For this review, take the finished solid that the model builds, in its own axes (mm). A direction names the side the tool comes from. Give positions to 0.01 mm unless a question says otherwise; leave off trailing zeros. Loops run counter-clockwise (first coordinate to the right, second up) from the corner with the lowest first, then second, coordinate; pieces in that order, holes last. Notation, with made-up numbers: (-13.5, -14) -> (39.5, -14) arc R24 ccw to (39.5, 8) -> close; hole circle Ø4 at (84, -24.5). An arc over 180 degrees is marked (long way). One line per question, with ' | ' between items. Start each with the question number.
(1) Consider section D-D (x = -9). Write out the cut boundary in (y, z).
(2) Consider section C-C (y = 0.25). Give the number of separate pieces and of enclosed holes in the cut face, and give its area (3 significant figures).
(3) Draft analysis for pull direction X (two halves, no side actions). For faces 1 (the flat face through (-17, 0, 0)), 2 (the cylindrical face through (-12, 0, -26)), 3 (the cylindrical face through (16.1, -0.02, -28.14)), state which applies: +X half, -X half, draft (parallel to the pull), parting line (faces both ways), or undercut.
(4) Insertion check: P1, Ø1.5, axis at x = 10.5, y = 0, coming from the +Z side; P2, Ø0.5, axis at x = 0, y = 0, coming from the +Z side. Each pin has a flat end and moves straight along its axis. Give the tip position at first contact, or say it passes through.
(5) Tool access review of faces 4 (the cylindrical face through (16.14, 0.02, 28.1)), 5 (the cylindrical face through (12, 0, -13)), 6 (the flat face through (1.5, 0, 27)): name each direction out of +Z, -Z, +X, -X, +Y, -Y from which nothing blocks a thin tool from reaching the whole face with its end or side.
(6) Consider section A-A (x = 3.5). Write out the cut boundary in (y, z).
(7) Consider section B-B (z = 0). Write out the cut boundary in (x, y), and give its area (3 significant figures).
(8) Wall thickness on probe 1 along X at (y, z) = (0.85, -17); probe 2 along Z at (x, y) = (2.5, 0.6); probe 3 along Z at (x, y) = (11, 0.45): over which ranges is each line inside the solid? List them lowest first.
from build123d import *

# Parameters (mm, degrees)
SKETCH1_W               = 34
SKETCH1_H               = 58
BOSS_EXTRUDE1_DEPTH     = 1.5
CUT_EXTRUDE1_DEPTH      = 34.648922717
CUT_EXTRUDE1_DEPTH_BACK = 34.648922717
CUT_EXTRUDE2_DEPTH      = 34.648922717
CUT_EXTRUDE2_DEPTH_BACK = 34.648922717
BOSS_EXTRUDE3_DEPTH     = 1.5
FILLET1_R               = 3


with BuildPart() as part:
    # Sketch1 → Boss-Extrude1 (new, symmetric)
    with BuildSketch(Plane(origin=(0, 0, 0), x_dir=(1, 0, 0), z_dir=(0, 1, 0))):
        Rectangle(SKETCH1_W, SKETCH1_H)
    extrude(amount=BOSS_EXTRUDE1_DEPTH, both=True)

    # Sketch3 → Cut-Extrude1 (cut, two sides: drawn at the far end of the back side and taken through both)
    with BuildSketch(Plane(origin=(0, 0, 0), x_dir=(1, 0, 0), z_dir=(0, 1, 0)).offset(-CUT_EXTRUDE1_DEPTH_BACK)):
        with BuildLine():
            Line((-13.5, 14.5), (-13.5, 24.5))
            ThreePointArc((-13.5, 24.5), (-12, 26), (-10.5, 24.5))
            Line((-10.5, 24.5), (-10.5, 14.5))
            ThreePointArc((-10.5, 14.5), (-12, 13), (-13.5, 14.5))
        make_face()
        with BuildLine():
            Line((-13.5, -6.5), (-13.5, 3.5))
            ThreePointArc((-13.5, 3.5), (-12, 5), (-10.5, 3.5))
            Line((-10.5, 3.5), (-10.5, -6.5))
            ThreePointArc((-10.5, -6.5), (-12, -8), (-13.5, -6.5))
        make_face()
        with BuildLine():
            Line((13.5, -6.5), (13.5, 3.5))
            ThreePointArc((13.5, 3.5), (12, 5), (10.5, 3.5))
            Line((10.5, 3.5), (10.5, -6.5))
            ThreePointArc((10.5, -6.5), (12, -8), (13.5, -6.5))
        make_face()
        with BuildLine():
            Line((13.5, 14.5), (13.5, 24.5))
            ThreePointArc((13.5, 24.5), (12, 26), (10.5, 24.5))
            Line((10.5, 24.5), (10.5, 14.5))
            ThreePointArc((10.5, 14.5), (12, 13), (13.5, 14.5))
        make_face()
        with BuildLine():
            Line((-6, 24), (6, 24))
            ThreePointArc((6, 24), (7.414213562, 23.414213562), (8, 22))
            Line((8, 22), (8, -4))
            ThreePointArc((8, -4), (7.414213562, -5.414213562), (6, -6))
            Line((6, -6), (-6, -6))
            ThreePointArc((-6, -6), (-7.414213562, -5.414213562), (-8, -4))
            Line((-8, -4), (-8, 22))
            ThreePointArc((-8, 22), (-7.414213562, 23.414213562), (-6, 24))
        make_face()
    extrude(amount=CUT_EXTRUDE1_DEPTH + CUT_EXTRUDE1_DEPTH_BACK, mode=Mode.SUBTRACT)

    # Sketch5 → Cut-Extrude2 (cut, two sides: drawn at the far end of the back side and taken through both)
    with BuildSketch(Plane(origin=(0, 0, 0), x_dir=(1, 0, 0), z_dir=(0, 1, 0)).offset(-CUT_EXTRUDE2_DEPTH_BACK)):
        with BuildLine():
            Line((-1.5, -29), (1.5, -29))
            Line((1.5, -29), (1.5, -25))
            Line((1.5, -25), (2.85, -25))
            Line((2.85, -25), (2.85, -22.73))
            Line((2.85, -22.73), (1.5, -22.73))
            Line((1.5, -22.73), (1.5, -18))
            ThreePointArc((1.5, -18), (1.207106781, -17.292893219), (0.5, -17))
            Line((0.5, -17), (-0.5, -17))
            ThreePointArc((-0.5, -17), (-1.207106781, -17.292893219), (-1.5, -18))
            Line((-1.5, -18), (-1.5, -22.73))
            Line((-1.5, -22.73), (-2.85, -22.73))
            Line((-2.85, -22.73), (-2.85, -25))
            Line((-2.85, -25), (-1.5, -25))
            Line((-1.5, -25), (-1.5, -29))
        make_face()
    extrude(amount=CUT_EXTRUDE2_DEPTH + CUT_EXTRUDE2_DEPTH_BACK, mode=Mode.SUBTRACT)

    # Sketch8 → Boss-Extrude3 (add, symmetric)
    with BuildSketch(Plane(origin=(0, 0, 0), x_dir=(1, 0, 0), z_dir=(0, 1, 0))):
        with BuildLine():
            Line((-7.7, -29), (-5.2, -29))
            Line((-5.2, -29), (-5.2, -31.5))
            ThreePointArc((-5.2, -31.5), (-5.346446609, -31.853553391), (-5.7, -32))
            Line((-5.7, -32), (-7.2, -32))
            ThreePointArc((-7.2, -32), (-7.553553391, -31.853553391), (-7.7, -31.5))
            Line((-7.7, -31.5), (-7.7, -29))
        make_face()
        with BuildLine():
            Line((5.2, -29), (5.2, -31.5))
            ThreePointArc((5.2, -31.5), (5.346446609, -31.853553391), (5.7, -32))
            Line((5.7, -32), (7.2, -32))
            ThreePointArc((7.2, -32), (7.553553391, -31.853553391), (7.7, -31.5))
            Line((7.7, -31.5), (7.7, -29))
            Line((7.7, -29), (5.2, -29))
        make_face()
    extrude(amount=BOSS_EXTRUDE3_DEPTH, both=True)

    # Fillet1
    fillet1_edges = [part.edges().sort_by_distance(p)[0] for p in [
        (-17, 0, -29),
        (17, 0, -29),
        (17, 0, 29),
        (-17, 0, 29),
    ]]
    fillet(fillet1_edges, radius=FILLET1_R)


solid = part.part
A:
1) outline: (-1.5, -29) -> (1.5, -29) -> (1.5, 29) -> (-1.5, 29) -> close
2) separate pieces: 1 | enclosed holes: 5 | area: 1,310 mm^2
3) face 1: -X half | face 2: undercut | face 3: +X half
4) P1: stops at z = 29 | P2: stops at z = 17
5) face 4: +Z, +X, +Y, -Y | face 5: +Y, -Y | face 6: +Z, +Y, -Y
6) outline: (-1.5, -29) -> (1.5, -29) -> (1.5, -24) -> (-1.5, -24) -> close; (-1.5, 6) -> (1.5, 6) -> (1.5, 29) -> (-1.5, 29) -> close
7) outline: (-17, -1.5) -> (-13.5, -1.5) -> (-13.5, 1.5) -> (-17, 1.5) -> close; (-10.5, -1.5) -> (-8, -1.5) -> (-8, 1.5) -> (-10.5, 1.5) -> close; (8, -1.5) -> (10.5, -1.5) -> (10.5, 1.5) -> (8, 1.5) -> close; (13.5, -1.5) -> (17, -1.5) -> (17, 1.5) -> (13.5, 1.5) -> close | area: 36.0 mm^2
8) probe 1: x = -17 to -13.5, -10.5 to -8, 8 to 10.5, 13.5 to 17 | probe 2: z = -29 to -24, 6 to 22.73, 25 to 29 | probe 3: z = -29 to -25.62, -13.38 to -4.62, 7.62 to 29
